Read the model definition and answer for the solid it produces. Units are mm, in the model's axes. A direction names the side the tool comes from. Give positions to 0.01 mm unless a question says otherwise; leave off trailing zeros. Order: outer loops, then holes, each group sorted by start corner. A loop starts at its lowest first (then second) coordinate and runs counter-clockwise, first axis right, second up. Notation, with made-up numbers: (21.25, 73) - (54.25, 73) arc R16 ccw to (54.25, 80) - close; hole circle Ø10 at (-24, 3). An arc over 180 degrees is marked (long way). Use a Markdown table: item, result. Add a question column.
1. Flat-ended cylindrical pins translate along their axes: P1, Ø1.5, axis at x = 14, y = -9, coming from the +Z side; P2, Ø6, axis at y = 24, z = -8, coming from the +X side; P3, Ø8, axis at x = 8, y = 59.5, coming from the +Z side. Find the tip coordinate at first contact, or state that the pin passes through.
2. Which of the six approach directions +Z, -Z, +X, -X, +Y, -Y give full straight-line access (tool end or side, diameter ignored) to faces 1 (the cylindrical face through (-4.8, -0.9, -21.7)), 2 (the flat face through (0, 64.262, 16))?
3. For a pull along Y with two mould halves and no side action, classify faces 3 (the flat face through (0, 68.326, 0)), 4 (the flat face through (0, 61, 12.573)), 5 (the flat face through (0, -68.326, 0)) as released by +Y, released by -Y, zero draft, split by the parting line, or undercut.
4. Consider L1, parallel to Y at x = 1, z = 18; L2, parallel to X at y = 43, z = -0.5. Determine where each line is inside the solid, lowest interval first.
5. A cutting plane is placed at A-A on y = 28.5. Determine the outline of the cut face in (x, z) (3 decimals), and give its area (3 significant figures).
```python
from build123d import *

# Parameters (mm, degrees)
F0_R     = 22.225
F1_DEPTH = 68.326
F2_SIZE  = 1.524
F3_W     = 7.112
F3_H     = 19.304
F4_DEPTH = 25.4


with BuildPart() as f1:
    # F0 (on Front) → F1 (new body, symmetric)
    with BuildSketch(Plane.XZ):
        Circle(F0_R)
    extrude(amount=F1_DEPTH, both=True)

    # F2
    f2_edges = [f1.edges().sort_by_distance(p)[0] for p in [
        (-22.225, -68.326, 0),
        (-22.225, 68.326, 0),
    ]]
    chamfer(f2_edges, length=F2_SIZE)

    # F3 (on Right) → F4 (cut, symmetric)
    with BuildSketch(Plane.YZ):
        with Locations((60.706, 22.225)):
            Rectangle(F3_W, F3_H)
    extrude(amount=F4_DEPTH, both=True, mode=Mode.SUBTRACT)


solid = f1.part
```
Output values:
| question | item | result |
|---|---|---|
| 1 | P1 | z = 17.84 |
| 1 | P2 | x = 21.66 |
| 1 | P3 | z = 21.71 |
| 2 | face 1 | +Y, -Y |
| 2 | face 2 | +Z, +X, -X |
| 3 | face 3 | released by +Y |
| 3 | face 4 | undercut |
| 3 | face 5 | released by -Y |
| 4 | L1 | -68.33 to 57.15, 64.26 to 68.33 |
| 4 | L2 | -22.22 to 22.22 |
| 5 | outline | circle Ø44.45 at (0, 0) |
| 5 | area | 1,550 mm² |
